Autodesk Inventor part; units mm, degrees
ref_plane "Arbeitsebene1" through (0, 10, -25) normal (0, 0, 1) x (1, 0, 0)
ref_plane "YZ Plane" through (0, 0, 0) normal (1, 0, 0) x (0, 1, 0)
ref_plane "XZ Plane" through (0, 0, 0) normal (0, 1, 0) x (-1, 0, 0)
sketch "Skizze1" plane through (0, 0, 0) normal (1, 0, 0) x (0, 1, 0)
  line L0 (0, 0) -> (0, -30)
  line L1 (0, -30) -> (40, -30)
  line L2 (40, -30) -> (40, -20)
  line L3 (40, -20) -> (10, -20)
  line L4 (10, -20) -> (10, 0)
  line L5 (10, 0) -> (0, 0)
  dimension "d0" = 40
  dimension "d1" = 30
  dimension "d2" = 10
  dimension "d3" = 10
extrude "Extrusion1" add sketch "Skizze1" along normal blind 30
ref_plane "Arbeitsebene1" through (0, 10, -25) normal (0, 0, 1) x (1, 0, 0)
sketch "Skizze2" plane through (0, 10, -25) normal (0, 0, 1) x (1, 0, 0)
  line L0 (0, -10) -> (0, 30)
  line L1 (0, 30) -> (30, 30)
  line L2 (30, -10) -> (30, 30)
  line L3 (0, 30) -> (30, 0) construction
  line L4 (30, 30) -> (0, 0) construction
  line L5 (0, 0) -> (30, 0) construction
  line L6 (5.2428, 15) -> (10.1214, 23.45)
  line L7 (10.1214, 23.45) -> (19.8786, 23.45)
  line L8 (19.8786, 23.45) -> (24.7572, 15)
  line L9 (24.7572, 15) -> (19.8786, 6.55)
  line L10 (19.8786, 6.55) -> (10.1214, 6.55)
  line L11 (10.1214, 6.55) -> (5.2428, 15)
  circle A0 centre (15, 15) radius 6
  dimension "d6" = 16.9
  dimension "d9" = 12
extrude "Extrusion2" cut sketch "Skizze2" along normal mid plane 3.6
extrude "Extrusion3" cut sketch "Skizze2" along normal mid plane 10 contours A0
sketch "Skizze3" plane through (0, 10, 0) normal (0, 1, 0) x (1, 0, 0)
  line L0 (0, 20) -> (0, 0)
  line L1 (0, 0) -> (30, 0)
  line L2 (30, 20) -> (30, 0)
  line L3 (0, 20) -> (30, 20)
  arc A0 (0, 20) -> (0, 0) centre (0, 10) ccw
  arc A1 (30, 0) -> (30, 20) centre (30, 10) ccw
  point P0 (0, 0)
extrude "Extrusion4" add sketch "Skizze3" against normal up to surface (10 mm away) contours L0 A0 | A1 L2
hole "Bohrung1" at (0, 10, -10) at (30, 10, -10) direction (0, -1, 0) diameter 3.4 end through all counterbore diameter 6.5 counterbore depth 3.4
fillet "Rundung1" radius 15 2 edges at (30, 40, -25) (0, 40, -25)
chamfer "Fasen1" distance 2 angle 45 9 edges at (15, 10, 0) (40, 10, -10) (-10, 10, -10) (30, 17.5001, -20) (25.6066, 35.6066, -20) (0, 17.5001, -20) (30, 12.5001, -30) (25.6066, 35.6066, -30) (0, 12.5001, -30)
chamfer "Fasen2" distance 2 angle 45 2 edges at (30, 10, -20) (0, 10, -20)
chamfer "Fasen3" distance 0.5 angle 45 6 edges at (0, 10, -13.25) (30, 10, -13.25) (0, 6.6, -11.7) (30, 6.6, -11.7) (9, 25, -20) (9, 25, -30)
chamfer "Fasen4" distance 2.2 angle 45 1 edges at (15, 10, -20)
properties part number "Sensorhalter_Portal" material "PC/ABS-Kunststoff"
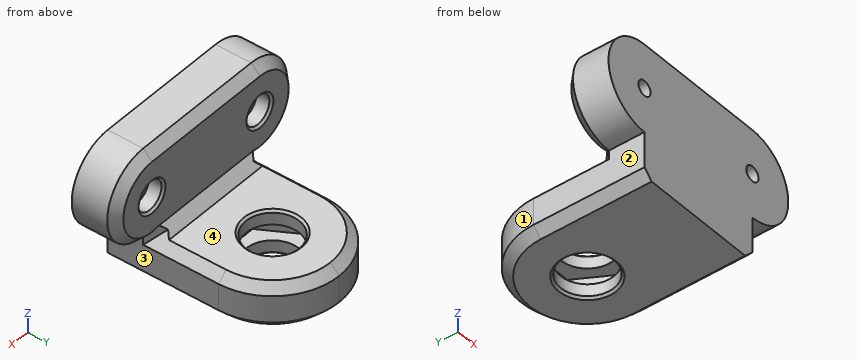
Part model, mm, in its own coordinate system. Face numbers are marked on the shaded views. A direction names the side the tool comes from. Round coordinates to 2 decimals unless told otherwise and drop trailing zeros. Order: outer loops, then holes, each group sorted by start corner. A loop starts at its lowest first (then second) coordinate and runs counter-clockwise, first axis right, second up. Notation, with made-up numbers: (53, -40) -> (91, -40) arc R26 ccw to (91, -26) -> close; hole circle Ø10 at (-38.5, 69). An arc over 180 degrees is marked (long way). Put each result on its own line as item: value.
Q1. Band-saw the part on B-B (y = 5.5). Give the cut face in (x, z), and give its area (3 significant figures).
From the geometry:
outline: (0, -28) -> (2, -30) -> (28, -30) -> (30, -28) -> (30, -20) arc R10 ccw to (30, 0) -> (0, 0) arc R10 ccw to (0, -20) -> close; hole circle Ø3.4 at (0, -10); hole circle Ø3.4 at (30, -10)
area: 1,190 mm2
Q2. Pin check, flat tips, straight feed: pin 1 Ø5 at (x, z) = (15, -10) entering from +Y; pin 2 Ø5 at (x, z) = (1, -9.5) entering from +Y; pin 3 Ø5 at (x, z) = (33.5, -17.5) entering from -Y; pin 4 Ø12 at (y, z) = (15, -22.5) entering from +X. Stop position of each tip, or through.
From the geometry:
pin 1: stops at y = 10
pin 2: stops at y = 9.87
pin 3: stops at y = 0
pin 4: stops at x = 30
Q3. Tool access for the marked faces 1, 2, 3 and 4: list every direction of +Z, -Z, +X, -X, +Y, -Y with a clear straight run to the whole face (end or side of a thin tool).
From the geometry:
face 1: +Z, -Z, -X, +Y
face 2: -Z, -X, +Y, -Y
face 3: -Z, +X, +Y, -Y
face 4: +Z, +X, -X, +Y
Q4. Band-saw the part on C-C (y = 15.5). Give the cut face in (x, z), and give its area (3 significant figures).
From the geometry:
outline: (0, -28) -> (2, -30) -> (28, -30) -> (30, -28) -> (30, -22) -> (28, -20) -> (2, -20) -> (0, -22) -> close
area: 292 mm2
Q5. Wall check: line 1 (X direction, y = 3.5, z = -10); line 2 (X direction, y = 8.8, z = -10); line 3 (X direction, y = 2, z = -24). Give the ranges that are in metal, low to high. Write a range as [from, to].
From the geometry:
line 1: x = [-10, -1.7], [1.7, 28.3], [31.7, 40]
line 2: x = [-9.2, -3.25], [3.25, 26.75], [33.25, 39.2]
line 3: x = [0, 30]
